```python
from build123d import *

# Parameters (mm, degrees)
F1_DEPTH = 6.35
F2_R     = 5.08


with BuildPart() as f1:
    # F0 (on Front) → F1 (new body)
    with BuildSketch(Plane.XZ):
        with BuildLine():
            Line((-19.05, 50.8), (-19.05, 0))
            ThreePointArc((-19.05, 0), (0, -19.05), (19.05, 0))
            Line((19.05, 0), (19.05, 50.8))
            Line((19.05, 50.8), (-19.05, 50.8))
        make_face()
    extrude(amount=F1_DEPTH)

    # F2
    f2_edges = [f1.edges().sort_by_distance(p)[0] for p in [
        (19.05, -3.175, 50.8),
        (-19.05, -3.175, 50.8),
    ]]
    fillet(f2_edges, radius=F2_R)


solid = f1.part
```
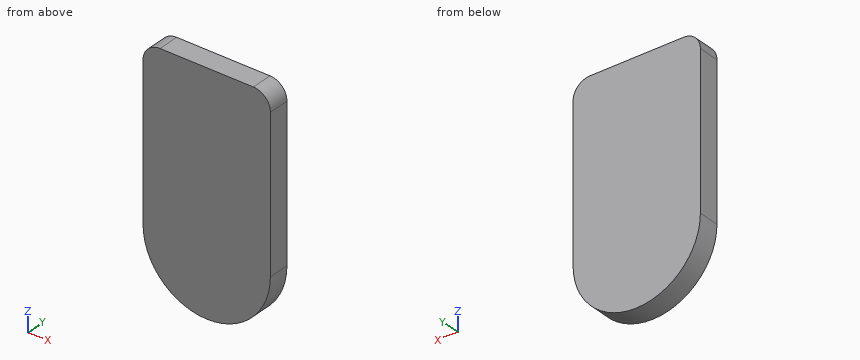
Verification items for the finished model (mm, model axes). Coordinates: 2 decimals unless noted, no trailing zeros. Loops run counter-clockwise (first coordinate to the right, second up) from the corner with the lowest first, then second, coordinate; pieces in that order, holes last. Notation, with made-up numbers: (75.5, -15.5) -> (100.5, -15.5) arc R32 ccw to (100.5, 14.5) -> close; hole circle Ø6 at (39.5, 70). An arc over 180 degrees is marked (long way). Answer in a Markdown table with one row per item. Add a question column.
1. Section check B-B, the plane x = 8. Enter the section's corners in (y, z), then the cut area to 3 significant figures.
2. Depth check by flat-ended pin: P1, Ø1.5, axis at x = 10.5, z = 39, coming from the +Y side. Enter the tip coordinate at first touch or a pass-through.
3. Material ranges on probe 1 along Z at (x, y) = (0, -3.75); probe 2 along X at (y, z) = (-4.5, 46); probe 3 along X at (y, z) = (-4.75, -7), recorded low to high. Write a range as [from, to].
4. Section check A-A, the plane y = -1.75. Enter the section's corners in (x, z), then the cut area to 3 significant figures.
5. Section check C-C, the plane x = -11. Enter the section's corners in (y, z), then the cut area to 3 significant figures.
Derived:
| question | item | result |
|---|---|---|
| 1 | outline | (-6.35, -17.29) -> (0, -17.29) -> (0, 50.8) -> (-6.35, 50.8) -> close |
| 1 | area | 432 mm² |
| 2 | P1 | stops at y = 0 |
| 3 | probe 1 | z = [-19.05, 50.8] |
| 3 | probe 2 | x = [-19.04, 19.04] |
| 3 | probe 3 | x = [-17.72, 17.72] |
| 4 | outline | (-19.05, 0) arc R19.05 ccw to (19.05, 0) -> (19.05, 45.72) arc R5.08 ccw to (13.97, 50.8) -> (-13.97, 50.8) arc R5.08 ccw to (-19.05, 45.72) -> close |
| 4 | area | 2,490 mm² |
| 5 | outline | (-6.35, -15.55) -> (0, -15.55) -> (0, 50.8) -> (-6.35, 50.8) -> close |
| 5 | area | 421 mm² |
